Read the model definition and answer for the solid it produces. Units are mm, in the model's axes. Coordinates: 2 decimals unless noted, no trailing zeros. Write each loop counter-clockwise with the first axis right and the second up, starting at its lowest first coordinate (ties: lowest second). Pieces come first, ordered by that corner, then holes.
(1) The part is cut by section D-D, the plane z = 1. Determine the outline of the cut face in (x, y), and give its area (3 significant figures).
(2) The part is cut by section C-C, the plane x = 0. Determine the outline of the cut face in (y, z), and give its area (3 significant figures).
(3) Determine the mould class of faces 1 (the cylindrical face through (-3.3, 24.8, 6.3)), 2 (the cylindrical face through (-1.05, -34.17, 6.26)), 3 (the cylindrical face through (1.97, 27.87, 6.26)), 4 (the flat face through (4, -25, 12.7)) for opening direction X: pulls with the +X half, pulls with the -X half, needs draft (parallel to the pull), parting line crosses it, or undercut.
(4) Straight lines are drawn through the part: line 1 along Y through (x, z) = (0, 4.75); line 2 along Y through (x, z) = (-3, 6.25); line 3 along X through (y, z) = (7.5, 3.75). For each, find the intervals that lie inside material, in ascending order.
(5) The part is cut by section B-B, the plane x = 7. Determine the outline of the cut face in (y, z).
(6) Given pin 1 (1 mm diameter, centred on x = -12, z = 7, fed in from -Y); pin 2 (3 mm diameter, centred on y = -14, z = 2.5, fed in from +X), each flat-ended and moving along its own axis, determine where each tip first touches the part or whether it passes through.
(7) The part is cut by section A-A, the plane y = 0. Determine the outline of the cut face in (x, z).
```python
from build123d import *

# Parameters (mm, degrees)
SKETCH1_R           = 27.94
SKETCH1_R_2         = 25.019
BOSS_EXTRUDE1_DEPTH = 12.7


with BuildPart() as part:
    # Sketch1 → Boss-Extrude1 (new body)
    with BuildSketch(Plane.XY):
        with BuildLine():
            ThreePointArc((-8.131862647, -26.730439762), (-9.164248984, -26.394320233), (-10.182796999, -26.018344399))
            ThreePointArc((-10.182796999, -26.018344399), (-1.113760176, -35.671945029), (8.539840454, -26.602908206))
            ThreePointArc((8.539840454, -26.602908206), (7.392494358, -26.944287468), (6.231578661, -27.236208021))
            ThreePointArc((6.231578661, -27.236208021), (-1.203026122, -34.165044546), (-8.131862647, -26.730439762))
        make_face()
        Circle(SKETCH1_R)
        Circle(SKETCH1_R_2, mode=Mode.SUBTRACT)
    extrude(amount=BOSS_EXTRUDE1_DEPTH)


solid = part.part
```
Computed:
1. outline: (-10.18, -26.02) arc R9.37 ccw to (8.54, -26.6) arc R27.94 ccw (long way) to start; hole circle Ø50.04 at (0, 0); hole (-8.13, -26.73) arc R7.19 ccw to (6.23, -27.24) arc R27.94 cw to start
1. area: 531 mm2
2. outline: (-35.64, 0) - (-34.11, 0) - (-34.11, 12.7) - (-35.64, 12.7) - close; (-27.94, 0) - (-25.02, 0) - (-25.02, 12.7) - (-27.94, 12.7) - close; (25.02, 0) - (27.94, 0) - (27.94, 12.7) - (25.02, 12.7) - close
2. area: 93.7 mm2
3. face 1: undercut
3. face 2: undercut
3. face 3: parting line crosses it
3. face 4: needs draft
4. line 1: y = -35.64 to -34.11, -27.94 to -25.02, 25.02 to 27.94
4. line 2: y = -35.42 to -33.87, -27.78 to -24.84, 24.84 to 27.78
4. line 3: x = -26.91 to -23.87, 23.87 to 26.91
5. outline: (-31.46, 0) - (-24.02, 0) - (-24.02, 12.7) - (-31.46, 12.7) - close; (24.02, 0) - (27.05, 0) - (27.05, 12.7) - (24.02, 12.7) - close
6. pin 1: stops at y = -25.46
6. pin 2: stops at x = 24.99
7. outline: (-27.94, 0) - (-25.02, 0) - (-25.02, 12.7) - (-27.94, 12.7) - close; (25.02, 0) - (27.94, 0) - (27.94, 12.7) - (25.02, 12.7) - close
